```python
from build123d import *

# Parameters (mm, degrees)
CROQUIS1_R                 = 62.36
CROQUIS1_R_2               = 42.36
SALIENTE_EXTRUIR1_DEPTH    = 20
CORTAR_EXTRUIR1_REACH      = 92.43
CORTAR_EXTRUIR1_END_RADIUS = 62.36
CROQUIS2_R                 = 1.25
MATRIZC1_COUNT             = 4


with BuildPart() as part:
    # Croquis1 → Saliente-Extruir1 (new body)
    with BuildSketch(Plane(origin=(0, 0, 0), x_dir=(1, 0, 0), z_dir=(0, 1, 0))):
        with Locations(Location((0, 0, 0), (0, 0, 270))):
            Circle(CROQUIS1_R)
        with Locations(Location((0, 0, 0), (0, 0, 270))):
            Circle(CROQUIS1_R_2, mode=Mode.SUBTRACT)
    extrude(amount=SALIENTE_EXTRUIR1_DEPTH)

    # Cortar-Extruir1: up to this cylinder (the profile starts inside it)
    cortar_extruir1_end = Plane(origin=(0, 10, 0), z_dir=(0, -1, 0)) * Cylinder(CORTAR_EXTRUIR1_END_RADIUS, 310.58, mode=Mode.PRIVATE)
    # Croquis2 → Cortar-Extruir1 (cut, up to the surface)
    with BuildSketch(Plane.XY, mode=Mode.PRIVATE) as cortar_extruir1_sk1:
        with Locations((0, 10)):
            Circle(CROQUIS2_R)
    cortar_extruir1_tool1 = extrude(cortar_extruir1_sk1.sketch, amount=-CORTAR_EXTRUIR1_REACH, mode=Mode.PRIVATE) & cortar_extruir1_end
    cortar_extruir1 = cortar_extruir1_tool1.solids().sort_by_distance((0, 10, 0))[0]
    add(cortar_extruir1, mode=Mode.SUBTRACT)

    # MatrizC1: Cortar-Extruir1 ×4 about axis
    matrizc1_axis = Axis((0, 20, 0), (0, 1, 0))
    for i in range(1, MATRIZC1_COUNT):
        add(cortar_extruir1.rotate(matrizc1_axis, i * 360 / MATRIZC1_COUNT), mode=Mode.SUBTRACT)


solid = part.part
```
The model under review builds one solid part; all positions refer to its coordinate system, in mm. Round coordinates to 2 decimals unless told otherwise and drop trailing zeros. Loops run counter-clockwise (first coordinate to the right, second up) from the corner with the lowest first, then second, coordinate; pieces in that order, holes last. Notation, with made-up numbers: (58.25, 24) - (111.25, 24) arc R29 ccw to (111.25, 51) - close; hole circle Ø5 at (-32, 5). An arc over 180 degrees is marked (long way). Write each question's results on one line, items separated by ' | '. Start each with the question number.
Q1. Take a section at B-B on x = -34. Give the boundary of the cut face in (y, z).
Q2. Take a section at C-C on y = 3. Give the boundary of the cut face in (x, z).
Q3. Take a section at A-A on z = -36.5. Give the boundary of the cut face in (x, y).
Q4. Wall thickness on line 1 along Y through (x, z) = (46, 0); line 2 along X through (y, z) = (14.5, 0): over which ranges is each line inside the solid? List them lowest first. Write a range as [from, to].
Q5. Draft analysis for pull direction Z (two halves, no side actions). For faces 1 (the flat face through (-13, 0, 41)), 2 (the cylindrical face through (-60.877, 9.86, -13.518)), 3 (the cylindrical face through (-41.353, 9.86, -9.183)), state which applies: pulls with the +Z half, pulls with the -Z half, needs draft (parallel to the pull), parting line crosses it, or undercut.
Q6. Insertion check: P1, Ø6, axis at x = 35, y = 14, coming from the -Z side; P2, Ø2, axis at x = 0, y = 10, coming from the +Z side; P3, Ø2, axis at x = 13.5, y = 4.5, coming from the +Z side; P4, Ø5, axis at x = 47.5, y = 16.5, coming from the -Z side. Each pin has a flat end and moves straight along its axis. Give the tip position at first contact, or say it passes through.
Data:
1) outline: (0, -52.28) - (20, -52.28) - (20, -25.27) - (0, -25.27) - close; (0, 25.27) - (20, 25.27) - (20, 52.28) - (0, 52.28) - close
2) outline: circle Ø124.72 at (0, 0); hole circle Ø84.72 at (0, 0)
3) outline: (-50.56, 0) - (-21.5, 0) - (-21.5, 20) - (-50.56, 20) - close; (21.5, 0) - (50.56, 0) - (50.56, 20) - (21.5, 20) - close
4) line 1: y = [0, 8.75], [11.25, 20] | line 2: x = [-62.36, -42.36], [42.36, 62.36]
5) face 1: needs draft | face 2: parting line crosses it | face 3: undercut
6) P1: stops at z = -53.52 | P2: passes through | P3: stops at z = 61.09 | P4: stops at z = -43.17
